```python
from build123d import *

# Parameters (mm, degrees)
SKETCH_1_W               = 110
SKETCH_1_H               = 57
SKETCH_1_R               = 8.5
SKETCH_1_R_2             = 2.5
EXTRUDE_1_DEPTH          = 5
SKETCH_2_W               = 5
SKETCH_2_H               = 10
EXTRUDE_2_DEPTH          = 5
PATTERN_LINEAR_1_COUNT   = 3
PATTERN_LINEAR_1_PITCH   = 20
MIRROR_1_COPY_1_SKETCH_W = 5
MIRROR_1_COPY_1_SKETCH_H = 10
MIRROR_1_COPY_1_DEPTH    = 5
MIRROR_1_COPY_2_SKETCH_W = 5
MIRROR_1_COPY_2_SKETCH_H = 10
MIRROR_1_COPY_2_DEPTH    = 5
SKETCH_3_W               = 10
SKETCH_3_H               = 5
EXTRUDE_3_DEPTH          = 5
PATTERN_LINEAR_2_COUNT   = 3
PATTERN_LINEAR_2_PITCH   = 20
PATTERN_LINEAR_3_COUNT   = 3
PATTERN_LINEAR_3_PITCH   = 20


with BuildPart() as part:
    # 스케치1 → 보스-돌출1 (new body)
    with BuildSketch(Plane.XY):
        Rectangle(SKETCH_1_W, SKETCH_1_H)
        with Locations((24, 2.5)):
            Circle(SKETCH_1_R, mode=Mode.SUBTRACT)
        with Locations((-24, 2.5)):
            Circle(SKETCH_1_R, mode=Mode.SUBTRACT)
        with Locations((-42.384776311, 20.884776311)):
            Circle(SKETCH_1_R_2, mode=Mode.SUBTRACT)
        with Locations((-5.615223689, -15.884776311)):
            Circle(SKETCH_1_R_2, mode=Mode.SUBTRACT)
        with Locations((5.615223689, 20.884776311)):
            Circle(SKETCH_1_R_2, mode=Mode.SUBTRACT)
        with Locations((42.384776311, -15.884776311)):
            Circle(SKETCH_1_R_2, mode=Mode.SUBTRACT)
    extrude(amount=EXTRUDE_1_DEPTH)

    # 스케치2 → 보스-돌출2 (add)
    with BuildSketch(Plane.XY.offset(5)):
        with Locations((57.5, -23.5)):
            Rectangle(SKETCH_2_W, SKETCH_2_H)
    extrude_2 = extrude(amount=-EXTRUDE_2_DEPTH)

    # 선형 패턴1: 보스-돌출2 ×3
    with Locations(*[(0, i * PATTERN_LINEAR_1_PITCH, 0) for i in range(1, PATTERN_LINEAR_1_COUNT)]):
        add(extrude_2)

    # 대칭 복사1: 보스-돌출2 across plane
    add(extrude_2.mirror(Plane(origin=(0, 0, 0), x_dir=(0, 0, 1), z_dir=(1, 0, 0))))

    # 대칭 복사1 copy 1 sketch → 대칭 복사1 copy 1 (add)
    with BuildSketch(Plane(origin=(0, 20, 5), x_dir=(-1, 0, 0), z_dir=(0, 0, 1))):
        with Locations((57.5, 23.5)):
            Rectangle(MIRROR_1_COPY_1_SKETCH_W, MIRROR_1_COPY_1_SKETCH_H)
    extrude(amount=-MIRROR_1_COPY_1_DEPTH)

    # 대칭 복사1 copy 2 sketch → 대칭 복사1 copy 2 (add)
    with BuildSketch(Plane(origin=(0, 40, 5), x_dir=(-1, 0, 0), z_dir=(0, 0, 1))):
        with Locations((57.5, 23.5)):
            Rectangle(MIRROR_1_COPY_2_SKETCH_W, MIRROR_1_COPY_2_SKETCH_H)
    extrude(amount=-MIRROR_1_COPY_2_DEPTH)

    # 스케치3 → 보스-돌출3 (add)
    with BuildSketch(Plane.XY.offset(5)):
        with Locations((0, 31)):
            Rectangle(SKETCH_3_W, SKETCH_3_H)
    extrude_3 = extrude(amount=-EXTRUDE_3_DEPTH)

    # 선형 패턴2: 보스-돌출3 ×3
    with Locations(*[(i * PATTERN_LINEAR_2_PITCH, 0, 0) for i in range(1, PATTERN_LINEAR_2_COUNT)]):
        add(extrude_3)

    # 선형 패턴3: 보스-돌출3 ×3
    with Locations(*[(-i * PATTERN_LINEAR_3_PITCH, 0, 0) for i in range(1, PATTERN_LINEAR_3_COUNT)]):
        add(extrude_3)


solid = part.part
```
Could you check a few things on this model? Use its own coordinates, in mm. A direction names the side the tool comes from. Round coordinates to 2 decimals unless told otherwise and drop trailing zeros. Loops run counter-clockwise (first coordinate to the right, second up) from the corner with the lowest first, then second, coordinate; pieces in that order, holes last. Notation, with made-up numbers: (51.25, 6) -> (104.25, 6) arc R30 ccw to (104.25, 29) -> close; hole circle Ø7 at (-37, 21). An arc over 180 degrees is marked (long way). Put each result on its own line as item: value.
Q1. I want a section at B-B on x = 22.5. Write out the boundary of the cut face in (y, z).
Checks:
outline: (-28.5, 0) -> (-5.87, 0) -> (-5.87, 5) -> (-28.5, 5) -> close; (10.87, 0) -> (33.5, 0) -> (33.5, 5) -> (10.87, 5) -> close
Q2. I want a section at A-A on x = 6.5. Write out the boundary of the cut face in (y, z).
Checks:
outline: (-28.5, 0) -> (18.55, 0) -> (18.55, 5) -> (-28.5, 5) -> close; (23.22, 0) -> (28.5, 0) -> (28.5, 5) -> (23.22, 5) -> close
Q3. Which directions (+Z, -Z, +X, -X, +Y, -Y) give clear straight access to the entire face, cutting with the end or side of a thin tool? Please do faces 4 (the flat face through (-10, 28.5, 2)), 5 (the flat face through (57, 11.5, 3)), 6 (the flat face through (45, 31, 3)).
Checks:
face 4: +Z, -Z, +Y
face 5: +Z, -Z, +X
face 6: +Z, -Z, +X, +Y
Q4. Please list where these lines run through material, in increasing order: line 1 (X direction, y = 29, z = 4.1); line 2 (Y direction, x = -24, z = 2.4); line 3 (X direction, y = 3, z = 4.05). Write a range as from..to.
Checks:
line 1: -45..-35, -25..-15, -5..5, 15..25, 35..45
line 2: -28.5..-6, 11..33.5
line 3: -55..-32.49, -15.51..15.51, 32.49..55
Q5. For pin 1 Ø10 at (x, y) = (24, 2.5) entering from -Z; pin 2 Ø2.5 at (y, z) = (30.5, 3.5) entering from +X; pin 3 Ø2.5 at (y, z) = (25, 1.5) entering from +X; pin 4 Ø2.5 at (y, z) = (30.5, 2) entering from -X, each with a flat end and sliding along its axis, tell me the tip position at first contact or that it passes through.
Checks:
pin 1: through
pin 2: x = 45
pin 3: x = 55
pin 4: x = -45
Q6. I want a section at D-D on z = 1.1. Give the number of separate pieces and of enclosed holes in the cut face, and give its area (3 significant figures).
Checks:
separate pieces: 1
enclosed holes: 6
area: 6,290 mm2
Q7. I want a section at C-C on y = 25. Write out the boundary of the cut face in (x, z), and give its area (3 significant figures).
Checks:
outline: (-55, 0) -> (55, 0) -> (55, 5) -> (-55, 5) -> close
area: 550 mm2
Q8. Thinking about a two-plate mould opening in Y: for faces 1 (the cylindrical face through (44.694, -16.842, 2.465)), 2 (the flat face through (-15, 31, 3)), 3 (the flat face through (0, 33.5, 3)), which applies, pulls with the +Y half, pulls with the -Y half, needs draft (parallel to the pull), parting line crosses it, or undercut?
Checks:
face 1: undercut
face 2: needs draft
face 3: pulls with the +Y half
